Geometry check sheet. Reference: the model listing, model coordinates, mm. A direction names the side the tool comes from. Round coordinates to 2 decimals unless told otherwise and drop trailing zeros. Order: outer loops, then holes, each group sorted by start corner. A loop starts at its lowest first (then second) coordinate and runs counter-clockwise, first axis right, second up. Notation, with made-up numbers: M 42.25,78.5 L 73.25,78.5 A22 ccw 73.25,89.5 Z; hole C 82.25,-22 d5. An arc over 180 degrees is marked long. Answer as a JSON object with one key per item and string values. Group by question number.
```python
from build123d import *

# Parameters (mm, degrees)
EXTRUDE_1_DEPTH     = 130
CUT_EXTRUDE_1_DEPTH = 130
SKETCH_3_W          = 56.400423759
SKETCH_3_H          = 132.12352691
CUT_EXTRUDE_2_DEPTH = 130
SKETCH_4_R          = 20
CUT_EXTRUDE_4_DEPTH = 536.34382743


with BuildPart() as part:
    # 草图1 → 凸台-拉伸1 (new body)
    with BuildSketch(Plane(origin=(0, 0, 0), x_dir=(0, 0, -1), z_dir=(1, 0, 0))):
        Polygon((-117.413418414, 203.995173877), (12.586581586, 227.58810424), (50.05442381, -170.65323063), (-276.483750531, -434.798684306), (-283.977318976, -355.150417332), (-37.902557252, -116.282866203), align=None)
    extrude(amount=EXTRUDE_1_DEPTH)

    # 草图2 → 切除-拉伸1 (cut)
    with BuildSketch(Plane(origin=(0, -127.628376299, -103.242003565), x_dir=(1, 0, 0), z_dir=(0, -0.7774718436693089, -0.6289177468488591))):
        Polygon((130, 138.410940137), (80, 488.410940137), (130, 488.410940137), align=None)
        Polygon((50, 488.410940137), (0, 138.410940137), (0, 488.410940137), align=None)
    extrude(amount=-CUT_EXTRUDE_1_DEPTH, mode=Mode.SUBTRACT)

    # 草图3 → 切除-拉伸2 (cut)
    with BuildSketch(Plane(origin=(0, 218.119745355, 39.585261254), x_dir=(1, 0, 0), z_dir=(0, 0.9839277155275394, 0.17856721596294645))):
        with Locations((68.261248993, -13.037702829)):
            Rectangle(SKETCH_3_W, SKETCH_3_H)
    extrude(amount=-CUT_EXTRUDE_2_DEPTH, mode=Mode.SUBTRACT)

    # 草图4 → 切除-拉伸4 (cut, through all)
    with BuildSketch(Plane.ZY):
        with Locations((46.203978927, 166.178708675)):
            Circle(SKETCH_4_R)
    extrude(amount=-CUT_EXTRUDE_4_DEPTH, mode=Mode.SUBTRACT)


solid = part.part
```
1) Release check for a two-part mould opening along Z. For faces 4 (the flat face through (112.996, 215.626, 53.323)), 5 (the cylindrical face through (113, 154.01, 30.33)), 6 (the flat face through (96.461, 155, 27)) record: +Z half, -Z half, draft (parallel to the pull), parting line (faces both ways), or undercut.
2) Sectioned sample at D-D (z = 208.5). Record the boundary of the cut face in (x, y).
3) Sectioned sample at A-A (z = 76). Record the boundary of the cut face in (x, y), then the cut area to 3 significant figures.
4) Set-up check for faces 1 (the flat face through (64.09, -210.848, 135.321)), 2 (the flat face through (19.8, -273.8, 134.8)), 3 (the flat face through (67.866, 87.766, 29.833)): record each of +Z, -Z, +X, -X, +Y, -Y from which the full face is reachable in a straight line by a thin tool's end or side.
5) Sectioned sample at C-C (y = -15). Record the boundary of the cut face in (x, z).
6) Go/stop test with flat-tipped pins: P1, Ø12, axis at x = 106, y = 81.5, coming from the -Z side; P2, Ø4, axis at x = 57, z = 9, coming from the -Y side; P3, Ø3, axis at x = 84, y = -194.5, coming from the +Z side. Record where each tip stops, or that it passes through.
7) Sectioned sample at B-B (x = 121). Record the boundary of the cut face in (y, z).
8) Thickness scan on line 1 along X through (y, z) = (170, -9); line 2 along Y through (x, z) = (46.5, -24.5); line 3 along Z through (x, y) = (41, -78.5). Record the ranges inside material, lowest first. Write a range as [from, to].
Final values:
{
 "1": {"face 4": "+Z half", "face 5": "undercut", "face 6": "draft"},
 "2": {"outline": "M 28.71,-281.88 L 37.51,-379.8 L 92.49,-379.8 L 101.29,-281.88 Z"},
 "3": {"outline": "M 0,37.18 L 130,37.18 L 130,211.51 L 96.46,211.51 L 96.46,79.39 L 40.06,79.39 L 40.06,211.51 L 0,211.51 Z; M 2.44,-153.26 L 13.16,-272.62 L 116.84,-272.62 L 127.56,-153.26 Z", "area": "28,900 mm^2"},
 "4": {"face 1": "+Z, +X, -X", "face 2": "+Z, -X, -Y", "face 3": "+Z, +Y"},
 "5": {"outline": "M 0,-35.41 L 130,-35.41 L 130,63.05 L 0,63.05 Z"},
 "6": {"P1": "stops at z = -26.9", "P2": "stops at y = -220.04", "P3": "stops at z = 120.02"},
 "7": {"outline": "M -254.3,53.35 L -170.65,-50.05 L 227.59,-12.59 L 204,117.41 L -116.28,37.9 L -185.39,109.09 Z; hole C 166.18,46.2 d40"},
 "8": {"line 1": "x = [0, 40.06], [96.46, 130]", "line 2": "y = [-191.32, 97.63]", "line 3": "z = [-41.38, 47.28]"}
}
